Model file for the job. Use its own axes, mm. A direction names the side the tool comes from. Round coordinates to 2 decimals unless told otherwise and drop trailing zeros. Write each loop counter-clockwise with the first axis right and the second up, starting at its lowest first coordinate (ties: lowest second). Pieces come first, ordered by that corner, then holes. Notation, with made-up numbers: (57, -26.75) - (112, -26.75) arc R21 ccw to (112, -9.75) - close; hole circle Ø9 at (-28.5, -21). An arc over 180 degrees is marked (long way). One line per item, written item: value.
Autodesk Inventor part; units mm, degrees
ref_plane "YZ Plane" through (0, 0, 0) normal (1, 0, 0) x (0, 1, 0)
ref_plane "XZ Plane" through (0, 0, 0) normal (0, 1, 0) x (-1, 0, 0)
ref_plane "XY Plane" through (0, 0, 0) normal (0, 0, 1) x (1, 0, 0)
sketch "Эскиз1" plane through (0, 0, 0) normal (0, 0, 1) x (1, 0, 0)
  line L0 (0, -0.6) -> (0, 3.6)
  line L1 (0, 0) -> (0, 3)
  line L2 (-24.75, 3) -> (24.75, 3)
  line L3 (-26.95, 0) -> (26.95, 0)
  line L4 (-24.75, 3) -> (-26.95, 0)
  line L5 (24.75, 3) -> (26.95, 0)
  line L6 (-25.85, 1.5) -> (25.85, 1.5)
  dimension "d1" = 3
  dimension "d3" = 49.5
  dimension "d4" = 53.9
extrude "Выдавливание1" add sketch "Эскиз1" along normal blind 90 contours L3 L4 L6 L0 | L0 L6 L5 L3
sketch "Эскиз2" plane through (-25.85, 1.5, 0) normal (0, 1, 0) x (1, 0, 0)
  line L0 (-1.1, 0) -> (52.8, 0)
  line L1 (20.85, 0) -> (30.85, 0)
  line L2 (30.85, 0) -> (30.85, -3)
  line L3 (30.85, -3) -> (20.85, -3)
  line L4 (20.85, -3) -> (20.85, 0)
  line L5 (25.85, 18) -> (25.85, -108)
  point P0 (25.85, 0)
  dimension "d7" = 10
  dimension "d8" = 3
extrude "Выдавливание2" add sketch "Эскиз2" along normal blind 2
fillet "Сопряжение1" radius 1 4 edges at (5, 2.5, 3) (5, 2.5, 0) (-5, 2.5, 3) (-5, 2.5, 0)
sketch "Эскиз7" plane through (-25.85, 1.5, 90) normal (0, 1, 0) x (1, 0, 0)
  line L0 (0, 90) -> (-1.1, 90)
  line L1 (45.7625, 90) -> (45.7625, 0) construction
  line L2 (45.7625, 0) -> (5.9375, 0) construction
  line L3 (5.9375, 0) -> (5.9375, 90) construction
  line L4 (5.9375, 90) -> (45.7625, 90) construction
  line L5 (51.7, 0) -> (0, 0)
  line L6 (-1.1, 0) -> (52.8, 0)
  line L7 (21.9773, 55.1118) -> (20.1462, 52.0958)
  line L8 (20.1462, 52.0958) -> (24.3419, 45.1851)
  line L9 (21.9773, 55.1118) -> (34.0311, 55.1118)
  line L10 (34.0311, 55.1118) -> (28.0042, 45.1851)
  line L11 (28.0042, 45.1851) -> (24.3419, 45.1851)
  line L12 (20.1462, 52.0958) -> (28.5377, 52.0958)
  line L13 (28.5377, 52.0958) -> (24.3419, 45.1851)
  line L14 (30.8592, 45.1851) -> (36.522, 45.1851)
  line L15 (36.522, 45.1851) -> (33.6906, 49.8437)
  line L16 (33.6906, 49.8437) -> (30.8592, 45.1851)
  line L17 (33.6906, 49.8437) -> (33.6906, 45.1851) construction
  line L18 (24.3419, 45.1851) -> (24.3419, 52.0958) construction
  line L19 (28.0042, 45.1851) -> (28.0042, 55.1118) construction
  line L20 (21.9773, 35.2585) -> (20.1462, 38.2745)
  line L21 (20.1462, 38.2745) -> (24.3419, 45.1851)
  line L22 (21.9773, 35.2585) -> (34.0311, 35.2585)
  line L23 (34.0311, 35.2585) -> (28.0042, 45.1851)
  line L24 (20.1462, 38.2745) -> (28.5377, 38.2745)
  line L25 (28.5377, 38.2745) -> (24.3419, 45.1851)
  line L26 (36.522, 45.1851) -> (33.6906, 40.5265)
  line L27 (33.6906, 40.5265) -> (30.8592, 45.1851)
  line L28 (33.6906, 40.5265) -> (33.6906, 45.1851) construction
  line L29 (24.3419, 45.1851) -> (24.3419, 38.2745) construction
  line L30 (28.0042, 45.1851) -> (28.0042, 35.2585) construction
  point P0 (25.85, 90)
  point P1 (51.7, 90)
  point P2 (25.85, 0)
emboss "Рельеф1" sketch "Эскиз7" operation cut depth 0.4 direction (0, -1, 0) contours L12 L13 L8 | L11 L23 L22 L20 L24 L25 | L14 L26 L27
sketch "Эскиз8" plane through (-25.85, 1.5, 90) normal (0, 1, 0) x (1, 0, 0)
  line L0 (30.8592, 45.1851) -> (36.522, 45.1851)
  line L1 (33.6906, 40.5265) -> (30.8592, 45.1851)
  line L2 (36.522, 45.1851) -> (33.6906, 40.5265)
  line L3 (24.3419, 45.1851) -> (28.0042, 45.1851)
  line L4 (28.5377, 38.2745) -> (24.3419, 45.1851)
  line L5 (20.1462, 38.2745) -> (28.5377, 38.2745)
  line L6 (21.9773, 35.2585) -> (20.1462, 38.2745)
  line L7 (34.0311, 35.2585) -> (21.9773, 35.2585)
  line L8 (28.0042, 45.1851) -> (34.0311, 35.2585)
  line L9 (20.1462, 52.0958) -> (28.5377, 52.0958)
  line L10 (24.3419, 45.1851) -> (20.1462, 52.0958)
  line L11 (28.5377, 52.0958) -> (24.3419, 45.1851)
  line L12 (33.6906, 49.8437) -> (30.8592, 45.1851)
  line L13 (36.522, 45.1851) -> (33.6906, 49.8437)
  line L14 (28.5377, 52.0958) -> (24.3419, 45.1851)
  line L15 (20.1462, 52.0958) -> (28.5377, 52.0958)
  line L16 (21.9773, 55.1118) -> (20.1462, 52.0958)
  line L17 (34.0311, 55.1118) -> (21.9773, 55.1118)
  line L18 (28.0042, 45.1851) -> (34.0311, 55.1118)
  line L19 (20.1462, 38.2745) -> (28.5377, 38.2745)
  line L20 (24.3419, 45.1851) -> (20.1462, 38.2745)
  line L21 (28.5377, 38.2745) -> (24.3419, 45.1851)
  point P0 (25.85, 90)
extrude "Выдавливание3" cut sketch "Эскиз8" against normal blind 0.2 contours L12 L13 L0 | L11 L9 L16 L17 L18 L3 | L4 L5 L20
properties part number "cover2_3DПЕЧАТЬ"
1. Drop flat-ended pins along their axis: pin 1 (5 mm diameter, centred on x = 7.5, z = 42.5, fed in from +Y); pin 2 (0.6 mm diameter, centred on x = 0.5, y = 3, fed in from +Z). Give the stop position or say it passes through.
Report:
pin 1: y = 1.5
pin 2: z = 3
2. Band-saw the part on C-C on x = 9.5. Write the cut outline in (y, z).
Report:
outline: (0, 0) - (1.5, 0) - (1.5, 42.89) - (1.3, 42.89) - (1.3, 44.81) - (1.1, 44.81) - (1.1, 46.74) - (1.5, 46.74) - (1.5, 90) - (0, 90) - close
3. Wall check: probe 1 along Y at (x, z) = (-15, 37.5); probe 2 along Y at (x, z) = (2, 45); probe 3 along Z at (x, y) = (2, 2.4). Give the ranges that are in metal, low to high. Write a range as [from, to].
Report:
probe 1: [0, 1.5]
probe 2: [0, 1.1]
probe 3: [0, 3]
4. Band-saw the part on D-D on x = -22. Write the cut outline in (y, z), plus the area to 3 significant figures.
Report:
outline: (0, 0) - (1.5, 0) - (1.5, 90) - (0, 90) - close
area: 135 mm²
5. Band-saw the part on A-A on y = 2.35. Write the cut outline in (x, z).
Report:
outline: (-5, 1) arc R1 ccw to (-4, 0) - (4, 0) arc R1 ccw to (5, 1) - (5, 2) arc R1 ccw to (4, 3) - (-4, 3) arc R1 ccw to (-5, 2) - close
6. Tool access for faces 1 (the face through (0, 3.5, 1)), 2 (the face through (5.125, 1.303, 49.709)): list every direction of +Z, -Z, +X, -X, +Y, -Y with a clear straight run to the whole face (end or side of a thin tool).
Report:
face 1: +Z, -Z, +X, -X, +Y
face 2: +Y
7. Band-saw the part on B-B on z = 46. Write the cut outline in (x, y).
Report:
outline: (-26.95, 0) - (26.95, 0) - (25.85, 1.5) - (9.95, 1.5) - (9.95, 1.1) - (5.73, 1.1) - (5.73, 1.5) - (2.87, 1.5) - (2.87, 1.1) - (-0.79, 1.1) - (-0.79, 1.3) - (-2.23, 1.3) - (-2.23, 1.5) - (-25.85, 1.5) - close
8. Mould opens along Z. For faces 3 (the face through (9.236, 1.303, 47.177)), 4 (the face through (6.4, 1.3, 47.1)), 5 (the face through (0, 2, 3)), 6 (the face through (0, 0, 44)) say: released by +Z, released by -Z, zero draft, split by the parting line, or undercut.
Report:
face 3: undercut
face 4: undercut
face 5: released by +Z
face 6: zero draft
